from build123d import *

# Parameters (mm, degrees)
SKETCH1_R           = 4.7625
BOSS_EXTRUDE1_DEPTH = 268.2875


# Read off the part's stored shape, not the designer's step: #10-32 Tapped Hole1
with BuildPart() as part:
    # Sketch1 → Boss-Extrude1 (new, symmetric)
    with BuildSketch(Plane.XY):
        Circle(SKETCH1_R)
    extrude(amount=BOSS_EXTRUDE1_DEPTH, both=True)

    # #10-32 Tapped Hole1 outline → #10-32 Tapped Hole1 (revolve, cut)
    with BuildSketch(Plane.XZ):
        Polygon((2.0193, -256.25806), (0, -255.044742152), (0, -268.2875), (2.0193, -268.2875), align=None)
        Polygon((0, 268.2875), (0, 255.044742152), (2.0193, 256.25806), (2.0193, 268.2875), align=None)
    revolve(axis=Axis((0, 0, 0), (0, 0, 1)), mode=Mode.SUBTRACT)


solid = part.part
The model under review builds one solid part; all positions refer to its coordinate system, in mm. Coordinates: 2 decimals unless noted, no trailing zeros. Loops run counter-clockwise (first coordinate to the right, second up) from the corner with the lowest first, then second, coordinate; pieces in that order, holes last. Notation, with made-up numbers: M 4,-35 L 30,-35 A25 cw 30,-5 Z; hole C -34.75,70 d7. An arc over 180 degrees is marked long. Put each result on its own line as item: value. Start each with the question number.
Q1. Add section A-A (z = 231). Write out the cut boundary in (x, y) (1 decimal), and give its area (3 significant figures).
Q2. Clearance check with flat-ended pins moving along their axes: pin 1 (2.5 mm diameter, centred on x = 0, y = 0, fed in from +Z); pin 2 (2 mm diameter, centred on x = -3.5, z = 127, fed in from +Y); pin 3 (1 mm diameter, centred on x = 2, z = 60.5, fed in from +Y). State where each tip first meets the part, or that it passes through.
Q3. Wall thickness on line 1 (Y direction, x = 0, z = 262.75); line 2 (X direction, y = -0.5, z = -126); line 3 (Z direction, x = -0.75, y = -1.75): over which ranges is each line inside the solid? List them lowest first.
Answers:
1. outline: C 0,0 d9.5
1. area: 71.3 mm^2
2. pin 1: stops at z = 255.8
2. pin 2: stops at y = 4.05
2. pin 3: stops at y = 4.52
3. line 1: y = -4.76 to -2.02, 2.02 to 4.76
3. line 2: x = -4.74 to 4.74
3. line 3: z = -256.19 to 256.19
